```python
from build123d import *

# Parameters (mm, degrees)
SKETCH_1_W          = 775
SKETCH_1_H          = 95
EXTRUDE_1_DEPTH     = 3
SKETCH_2_W          = 775
SKETCH_2_H          = 3
EXTRUDE_2_DEPTH     = 17
SKETCH_3_R          = 3.5
CUT_EXTRUDE_1_DEPTH = 17
SKETCH_4_R          = 2.5
CUT_EXTRUDE_2_DEPTH = 17
FILLET_1_R          = 5
FILLET_2_R          = 2


with BuildPart() as part:
    # 스케치1 → 보스-돌출1 (new body)
    with BuildSketch(Plane.XY):
        with Locations((387.5, 47.5)):
            Rectangle(SKETCH_1_W, SKETCH_1_H)
    extrude(amount=EXTRUDE_1_DEPTH)

    # 스케치2 → 보스-돌출2 (add)
    with BuildSketch(Plane.XY.offset(3)):
        with Locations((387.5, 1.5)):
            Rectangle(SKETCH_2_W, SKETCH_2_H)
    extrude(amount=EXTRUDE_2_DEPTH)

    # 스케치3 → 컷-돌출1 (cut)
    with BuildSketch(Plane.XY.offset(3)):
        with Locations((107.5, 55)):
            Circle(SKETCH_3_R)
        with Locations((107.5, 20)):
            Circle(SKETCH_3_R)
        with Locations((387.5, 55)):
            Circle(SKETCH_3_R)
        with Locations((387.5, 20)):
            Circle(SKETCH_3_R)
        with Locations((667.5, 55)):
            Circle(SKETCH_3_R)
        with Locations((667.5, 20)):
            Circle(SKETCH_3_R)
    extrude(amount=-CUT_EXTRUDE_1_DEPTH, mode=Mode.SUBTRACT)

    # 스케치4 → 컷-돌출2 (cut)
    with BuildSketch(Plane(origin=(0, 3, 0), x_dir=(1, 0, 0), z_dir=(0, 1, 0))):
        with Locations(Location((60, -11.5, 0), (0, 0, 270))):
            Circle(SKETCH_4_R)
        with Locations(Location((715, -11.5, 0), (0, 0, 270))):
            Circle(SKETCH_4_R)
    extrude(amount=-CUT_EXTRUDE_2_DEPTH, mode=Mode.SUBTRACT)

    # 필렛1
    fillet_1_edges = [part.edges().sort_by_distance(p)[0] for p in [
        (387.5, 0, 0),
    ]]
    fillet(fillet_1_edges, radius=FILLET_1_R)

    # 필렛2
    fillet_2_edges = [part.edges().sort_by_distance(p)[0] for p in [
        (387.5, 3, 3),
    ]]
    fillet(fillet_2_edges, radius=FILLET_2_R)


solid = part.part
```
CAD build for the part. Positions are in the model's coordinates, mm. A direction names the side the tool comes from. Coordinates: 2 decimals unless noted, no trailing zeros. Write each loop counter-clockwise with the first axis right and the second up, starting at its lowest first coordinate (ties: lowest second). Pieces come first, ordered by that corner, then holes.
(1) Flat gauge pins, fed straight in: pin 1 (2 mm diameter, centred on x = 378.5, z = 16.5, fed in from +Y); pin 2 (6.5 mm diameter, centred on x = 107.5, y = 55, fed in from -Z); pin 3 (12 mm diameter, centred on x = 194, z = 10.5, fed in from +Y); pin 4 (1 mm diameter, centred on x = 409, z = 3, fed in from -Y). Where does each tip first touch, or does it go through?
(2) 3-axis set-ups, long thin cutter, end or side, ignore diameter. For faces 1 (the face through (382, 51, 3)), 2 (the face through (0, 40, 2)): which of +Z, -Z, +X, -X, +Y, -Y reach the whole face in a straight line?
(3) Drill centre lines: probe 1 along X at (y, z) = (2.2, 11.5); probe 2 along Y at (x, z) = (667.5, 1.15); probe 3 along Z at (x, y) = (458, 54.5). Where is each one in solid material? Low to high.
(4) Cut at A-A, the plane x = 575. List the corners of the cut face in (y, z), and give its area (3 significant figures).
(5) Cut at B-B, the plane y = 35. List the corners of the cut face in (x, z), and give its area (4 significant figures).
Geometry says:
1. pin 1: stops at y = 3
1. pin 2: passes through
1. pin 3: stops at y = 3.06
1. pin 4: stops at y = 0.23
2. face 1: +Z, +X, -X, +Y
2. face 2: +Z, -Z, -X, +Y, -Y
3. probe 1: x = 0 to 57.5, 62.5 to 712.5, 717.5 to 775
3. probe 2: y = 1.81 to 16.5, 23.5 to 51.5, 58.5 to 95
3. probe 3: z = 0 to 3
4. outline: (0, 5) arc R5 ccw to (5, 0) - (95, 0) - (95, 3) - (5, 3) arc R2 cw to (3, 5) - (3, 20) - (0, 20) - close
4. area: 331 mm2
5. outline: (0, 0) - (775, 0) - (775, 3) - (0, 3) - close
5. area: 2,325 mm2
